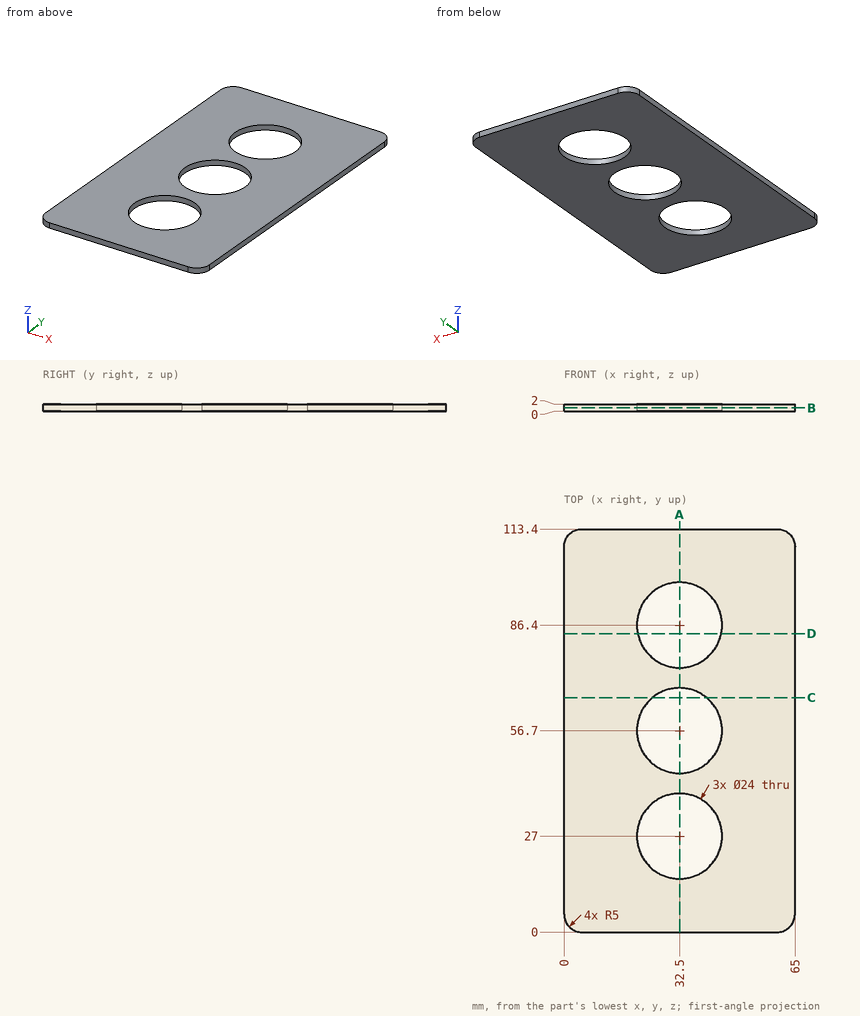
Could you check a few things on this drawing? It's one solid part, dimensions in mm from its lowest x, y, z. Round coordinates to 2 decimals unless told otherwise and drop trailing zeros. Order: outer loops, then holes, each group sorted by start corner. A loop starts at its lowest first (then second) coordinate and runs counter-clockwise, first axis right, second up. Notation, with made-up numbers: M -33,32 L 18,32 A9 ccw 18,40 Z; hole C -21.5,52.25 d1. An arc over 180 degrees is marked long. One line per item, written item: value.
(1) Imagine slicing it at D-D (y = 84). Write out the boundary of the cut face in (x, z), and give its area (3 significant figures).
Ans:
outline: M 0,0 L 20.74,0 L 20.74,2 L 0,2 Z; M 44.26,0 L 65,0 L 65,2 L 44.26,2 Z
area: 83.0 mm^2
(2) Imagine slicing it at C-C (y = 66). Write out the boundary of the cut face in (x, z), and give its area (3 significant figures).
Ans:
outline: M 0,0 L 24.92,0 L 24.92,2 L 0,2 Z; M 40.08,0 L 65,0 L 65,2 L 40.08,2 Z
area: 99.7 mm^2
(3) I need wall thicknesses on line 1 along Y through (x, z) = (32.5, 1.15); line 2 along Y through (x, z) = (38, 1.25); line 3 along X through (y, z) = (65, 1.8). Which ranges of each line are inside material? Lowest first, please. Write a range as from..to.
Ans:
line 1: y = 0..15, 39..44.7, 68.7..74.4, 98.4..113.4
line 2: y = 0..16.33, 37.67..46.03, 67.37..75.73, 97.07..113.4
line 3: x = 0..23.83, 41.17..65
(4) Imagine slicing it at B-B (z = 0.9). Write out the boundary of the cut face in (x, y).
Ans:
outline: M 0,5 A5 ccw 5,0 L 60,0 A5 ccw 65,5 L 65,108.4 A5 ccw 60,113.4 L 5,113.4 A5 ccw 0,108.4 Z; hole C 32.5,27 d24; hole C 32.5,56.7 d24; hole C 32.5,86.4 d24
(5) Imagine slicing it at A-A (x = 32.5). Write out the boundary of the cut face in (y, z).
Ans:
outline: M 0,0 L 15,0 L 15,2 L 0,2 Z; M 39,0 L 44.7,0 L 44.7,2 L 39,2 Z; M 68.7,0 L 74.4,0 L 74.4,2 L 68.7,2 Z; M 98.4,0 L 113.4,0 L 113.4,2 L 98.4,2 Z
